Answer from the drawing. Dimensions are ordinates in mm from the lowest x, y and z of the part. A direction names the side the tool comes from. Give positions to 0.01 mm unless a question says otherwise; leave off trailing zeros. Loops run counter-clockwise (first coordinate to the right, second up) from the corner with the lowest first, then second, coordinate; pieces in that order, holes last.
Item 1: Section B-B, the plane z = 4.5 is taken. Give the vertices of the cut face in (x, y) (1 decimal), and give its area (3 significant figures).
Item 2: Consider line 1 along X through (y, z) = (7.5, 5.75); line 2 along X through (y, z) = (9, 5.5); line 3 along Y through (x, z) = (5.5, 5.5) (1 decimal). Determine where each line is inside the solid, lowest interval first.
Item 3: A tool of negligible diameter and unlimited length cuts with its end or side. For the marked faces 1 and 2, from which of +Z, -Z, +X, -X, +Y, -Y can it reach the whole face along a straight path? Write none if from no direction.
Item 4: The mould has two halves that part along Y. Classify the marked faces 3, 4 and 5: pulls with the +Y half, pulls with the -Y half, needs draft (parallel to the pull), parting line crosses it, or undercut.
Item 5: Section D-D, the plane y = 9.25 is taken. Give the number of separate pieces and of enclosed holes in the cut face, and give its area (3 significant figures).
Item 6: Section A-A, the plane y = 6.5 is taken. Give the vertices of the cut face in (x, z), and give its area (3 significant figures).
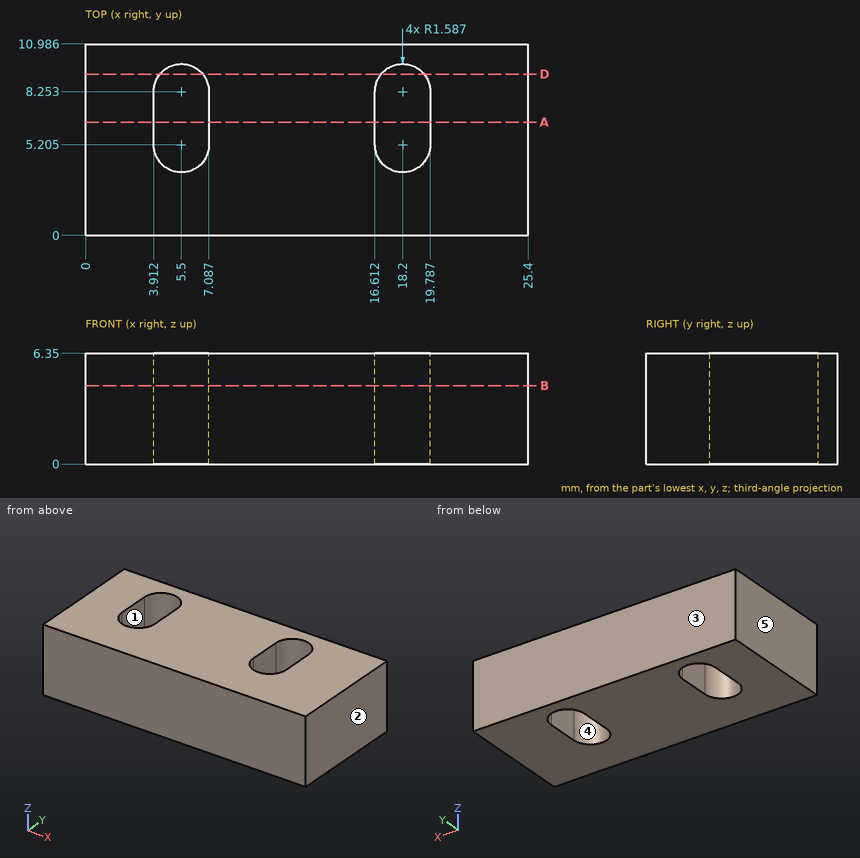
Worked answers:
1. outline: (0, 0) - (25.4, 0) - (25.4, 11) - (0, 11) - close; hole (3.9, 5.2) arc R1.6 ccw to (7.1, 5.2) - (7.1, 8.3) arc R1.6 ccw to (3.9, 8.3) - close; hole (16.6, 5.2) arc R1.6 ccw to (19.8, 5.2) - (19.8, 8.3) arc R1.6 ccw to (16.6, 8.3) - close
1. area: 244 mm2
2. line 1: x = 0 to 3.91, 7.09 to 16.61, 19.79 to 25.4
2. line 2: x = 0 to 4.1, 6.9 to 16.8, 19.6 to 25.4
2. line 3: y = 0 to 3.6, 9.8 to 11
3. face 1: +Z, -Z
3. face 2: +Z, -Z, +X, +Y, -Y
4. face 3: pulls with the +Y half
4. face 4: undercut
4. face 5: needs draft
5. separate pieces: 3
5. enclosed holes: 0
5. area: 130 mm2
6. outline: (0, 0) - (3.91, 0) - (3.91, 6.35) - (0, 6.35) - close; (7.09, 0) - (16.61, 0) - (16.61, 6.35) - (7.09, 6.35) - close; (19.79, 0) - (25.4, 0) - (25.4, 6.35) - (19.79, 6.35) - close
6. area: 121 mm2
